```python
from build123d import *

# Parameters (mm, degrees)
SKETCH_W        = 54
SKETCH_H        = 26
SKETCH_R        = 1.1
SKETCH_W_2      = 9
SKETCH_H_2      = 6.2
PAD_DEPTH       = 2
SKETCH001_W     = 54
SKETCH001_H     = 28
SKETCH001_W_2   = 52
SKETCH001_H_2   = 26
PAD001_DEPTH    = 10
PAD002_DEPTH    = 52
POCKET_DEPTH    = 54.001
SKETCH004_W     = 54
SKETCH004_H     = 28
SKETCH004_W_2   = 52
SKETCH004_H_2   = 26
PAD003_DEPTH    = 12
SKETCH005_W     = 54
SKETCH005_H     = 28
PAD004_DEPTH    = 1
POCKET001_DEPTH = 5
CHAMFER_SIZE    = 0.5
CHAMFER001_SIZE = 0.5
CHAMFER002_SIZE = 0.5
CHAMFER003_SIZE = 0.8
CHAMFER004_SIZE = 0.5


with BuildPart() as part:
    # Sketch → Pad (new body)
    with BuildSketch(Plane.XY):
        with Locations((27, 13)):
            Rectangle(SKETCH_W, SKETCH_H)
        with Locations((40.5, 13)):
            Circle(SKETCH_R, mode=Mode.SUBTRACT)
        with Locations((18.5, 13)):
            Rectangle(SKETCH_W_2, SKETCH_H_2, mode=Mode.SUBTRACT)
    extrude(amount=PAD_DEPTH)

    # Sketch001 (on Face11 of Pad) → Pad001 (join)
    with BuildSketch(Plane.XY.offset(2)):
        with Locations((27, 13)):
            Rectangle(SKETCH001_W, SKETCH001_H)
        with Locations((27, 13)):
            Rectangle(SKETCH001_W_2, SKETCH001_H_2, mode=Mode.SUBTRACT)
    extrude(amount=PAD001_DEPTH)

    # Sketch002 (on Face22 of Pad001) → Pad002 (join)
    with BuildSketch(Plane.YZ.offset(1)):
        Polygon((0, 2), (0, 3), (1, 2), align=None)
        Polygon((26, 2), (26, 3), (25, 2), align=None)
    extrude(amount=PAD002_DEPTH)

    # Sketch003 (on Face8 of Pad002) → Pocket (cut, through all)
    with BuildSketch(Plane.YZ.offset(54)):
        Polygon((-1, 2), (-1, 3), (0, 2), align=None)
        Polygon((27, 2), (27, 3), (26, 2), align=None)
    extrude(amount=-POCKET_DEPTH, mode=Mode.SUBTRACT)

    # Sketch004 (on Face17 of Pocket) → Pad003 (join)
    with BuildSketch(Plane.XY.offset(12)):
        with Locations((27, 13)):
            Rectangle(SKETCH004_W, SKETCH004_H)
        with Locations((27, 13)):
            Rectangle(SKETCH004_W_2, SKETCH004_H_2, mode=Mode.SUBTRACT)
    extrude(amount=PAD003_DEPTH)

    # Sketch005 (on Face22 of Pad003) → Pad004 (join)
    with BuildSketch(Plane.XY.offset(24)):
        with Locations((27, 13)):
            Rectangle(SKETCH005_W, SKETCH005_H)
    extrude(amount=PAD004_DEPTH)

    # Sketch006 (on Face26 of Pad004) → Pocket001 (cut)
    with BuildSketch(Plane(origin=(53, 0, 0), x_dir=(0, -1, 0), z_dir=(-1, 0, 0))):
        Polygon((-26, 24), (0, 24), (0, 3), (-1, 2), (-25, 2), (-26, 3), align=None)
    extrude(amount=-POCKET001_DEPTH, mode=Mode.SUBTRACT)

    # Chamfer
    chamfer_edges = [part.edges().sort_by_distance(p)[0] for p in [
        (54, -1, 24.5),
        (54, -1, 18),
        (54, -1, 7.5),
        (54, 27, 24.5),
        (54, 27, 18),
        (54, 27, 7.5),
        (54, -0.5, 2.5),
        (54, 26.5, 2.5),
        (0, 27, 7.5),
        (0, 27, 18),
        (0, 27, 24.5),
        (0, -1, 7.5),
        (0, -1, 18),
        (0, -1, 24.5),
    ]]
    chamfer(chamfer_edges, length=CHAMFER_SIZE)

    # Chamfer001
    chamfer001_edges = [part.edges().sort_by_distance(p)[0] for p in [
        (27, 27, 25),
        (0.25, 26.75, 25),
        (0, 13, 25),
        (0.25, -0.75, 25),
        (27, -1, 25),
        (53.75, -0.75, 25),
        (54, 13, 25),
        (53.75, 26.75, 25),
    ]]
    chamfer(chamfer001_edges, length=CHAMFER001_SIZE)

    # Chamfer002
    chamfer002_edges = [part.edges().sort_by_distance(p)[0] for p in [
        (27, 0, 24),
        (27, 26, 24),
        (1, 13, 24),
        (1, 26, 18),
        (1, 26, 7.5),
        (1, 0, 7.5),
        (1, 0, 18),
    ]]
    chamfer(chamfer002_edges, length=CHAMFER002_SIZE)

    # Chamfer003
    chamfer003_edges = [part.edges().sort_by_distance(p)[0] for p in [
        (0, 0, 1),
        (0, 13, 0),
        (0, 26, 1),
    ]]
    chamfer(chamfer003_edges, length=CHAMFER003_SIZE)

    # Chamfer004
    chamfer004_edges = [part.edges().sort_by_distance(p)[0] for p in [
        (27.4, 0, 0),
        (54, 13, 0),
        (27.4, 26, 0),
    ]]
    chamfer(chamfer004_edges, length=CHAMFER004_SIZE)


solid = part.part
```
Input: part model. Units: mm. Frame: model coordinates. A direction names the side the tool comes from. Coordinates: 2 decimals unless noted, no trailing zeros. Write each loop counter-clockwise with the first axis right and the second up, starting at its lowest first coordinate (ties: lowest second). Pieces come first, ordered by that corner, then holes. Notation, with made-up numbers: (70, 24.5) -> (80, 24.5) arc R19 ccw to (80, 39.5) -> close; hole circle Ø10 at (74, 11). An arc over 180 degrees is marked (long way). Write each question's results on one line, items separated by ' | '.
Item 1: Material intervals for probe 1 along Y at (x, z) = (22, 11.25); probe 2 along Y at (x, z) = (40.5, 1.05); probe 3 along Z at (x, y) = (12, 7.5), sorted ascending.
Conclusion:
probe 1: y = -1 to 0, 26 to 27 | probe 2: y = 0 to 11.9, 14.1 to 26 | probe 3: z = 0 to 2, 24 to 25
Item 2: Pin query (flat end, axial travel): pin 1 Ø1 at (x, z) = (19.5, 0.5) entering from -Y; pin 2 Ø1.8 at (x, z) = (15, 1) entering from +Y; pin 3 Ø1.6 at (x, z) = (20, 1.5) entering from +Y. Return the tip coordinate at first contact, or that it passes through.
Conclusion:
pin 1: stops at y = 0 | pin 2: stops at y = 26 | pin 3: stops at y = 26.3
Item 3: Section query B-B on x = 34. Return loops of the section in (y, z), plus the area to 3 significant figures.
Conclusion:
outline: (-1, 3) -> (0, 2) -> (0, 0.5) -> (0.5, 0) -> (25.5, 0) -> (26, 0.5) -> (26, 2) -> (27, 3) -> (27, 24.5) -> (26.5, 25) -> (-0.5, 25) -> (-1, 24.5) -> close; hole (0, 3) -> (1, 2) -> (25, 2) -> (26, 3) -> (26, 23.5) -> (25.5, 24) -> (0.5, 24) -> (0, 23.5) -> close | area: 124 mm^2
Item 4: Section query C-C on z = 20. Return loops of the section in (x, y).
Conclusion:
outline: (0, -0.5) -> (0.5, -1) -> (53.5, -1) -> (54, -0.5) -> (54, 0) -> (1.5, 0) -> (1, 0.5) -> (1, 25.5) -> (1.5, 26) -> (54, 26) -> (54, 26.5) -> (53.5, 27) -> (0.5, 27) -> (0, 26.5) -> close
Item 5: Mould query, pull axis Z, two halves, no side actions, for faces 4 (the flat face through (27, 26, 1)), 5 (the flat face through (27.1, 0.5, 2.5)), 6 (the flat face through (27.1, -0.5, 2.5)). Classes: +Z half, -Z half, draft (parallel to the pull), parting line (faces both ways), or undercut.
Conclusion:
face 4: draft | face 5: undercut | face 6: -Z half
Item 6: Section query D-D on x = 40.5. Return loops of the section in (y, z), plus the area to 3 significant figures.
Conclusion:
outline: (-1, 3) -> (0, 2) -> (0, 0.5) -> (0.5, 0) -> (11.9, 0) -> (11.9, 2) -> (1, 2) -> (0, 3) -> (0, 23.5) -> (0.5, 24) -> (25.5, 24) -> (26, 23.5) -> (26, 3) -> (25, 2) -> (14.1, 2) -> (14.1, 0) -> (25.5, 0) -> (26, 0.5) -> (26, 2) -> (27, 3) -> (27, 24.5) -> (26.5, 25) -> (-0.5, 25) -> (-1, 24.5) -> close | area: 119 mm^2
Item 7: Set-up query: faces 1 (the flat face through (27, 26, 13)), 2 (the flat face through (27, 27, 14)), 3 (the cylindrical face through (41.008, 12.024, 0.986)). Return all of +Z, -Z, +X, -X, +Y, -Y with unobstructed straight access to the full face (end or side cutting, diameter ignored); none if empty.
Conclusion:
face 1: +X | face 2: +Z, -Z, +X, -X, +Y | face 3: -Z
Item 8: Section query A-A on y = 13. Return loops of the section in (x, z).
Conclusion:
outline: (0, 0.8) -> (0.8, 0) -> (14, 0) -> (14, 2) -> (1, 2) -> (1, 23.5) -> (1.5, 24) -> (54, 24) -> (54, 24.5) -> (53.5, 25) -> (0.5, 25) -> (0, 24.5) -> close; (23, 0) -> (39.4, 0) -> (39.4, 2) -> (23, 2) -> close; (41.6, 0) -> (53.5, 0) -> (54, 0.5) -> (54, 2) -> (41.6, 2) -> close
